from build123d import *

# Parameters (mm, degrees)
F0_W     = 15
F0_H     = 10
F0_R     = 2
F1_DEPTH = 8.5
F2_W     = 2.25
F2_H     = 3.4951120354
F3_DEPTH = 25
F4_DEPTH = 6.5


with BuildPart() as f1:
    # F0 (on Top) → F1 (new body)
    with BuildSketch(Plane.XY):
        Rectangle(F0_W, F0_H)
        Circle(F0_R, mode=Mode.SUBTRACT)
    extrude(amount=F1_DEPTH)

    # F2 (on face) → F3 (cut)
    with BuildSketch(Plane.YZ.offset(7.5)):
        Polygon((5, 3), (2, 0), (5, 0), align=None)
        with Locations((3.875, 4.7475560177)):
            Rectangle(F2_W, F2_H)
        with Locations((-3.875, 4.7475560177)):
            Rectangle(F2_W, F2_H)
        Polygon((-5, 0), (-2, 0), (-5, 3), align=None)
    extrude(amount=-F3_DEPTH, mode=Mode.SUBTRACT)

    # F4 (cut): faces of the model
    f4_faces = [f1.faces().sort_by_distance(p)[0] for p in [
        (4.5185944257, 0, 0),
        (-4.5185944257, 0, 0),
    ]]
    extrude(f4_faces, amount=-F4_DEPTH, mode=Mode.SUBTRACT)


solid = f1.part
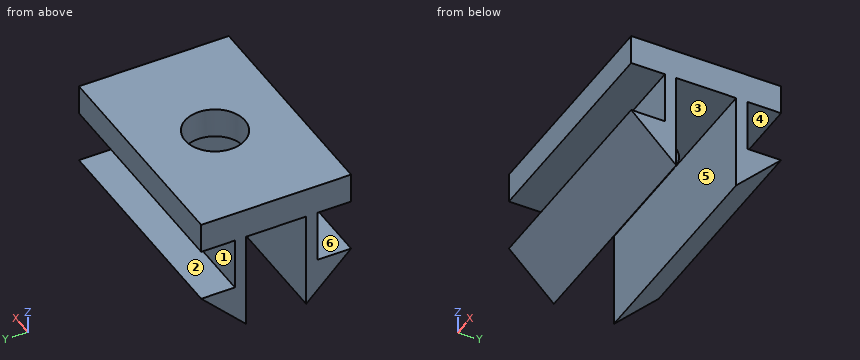
Here's how the part is built. I have some questions about the finished solid (model axes, mm). Face numbers are marked on the shaded views. A direction names the side the tool comes from. Coordinates: 2 decimals unless noted, no trailing zeros. Write each loop counter-clockwise with the first axis right and the second up, starting at its lowest first coordinate (ties: lowest second). Pieces come first, ordered by that corner, then holes.
Item 1: On a 3-axis mill with a long thin cutter (end or side, diameter ignored), from which of +Z, -Z, +X, -X, +Y, -Y can I reach the whole of each face in a straight line? I mean the marked faces 4, 5 and 6. Say none if no direction works.
Item 2: If I drill on line 1 (Y direction, x = 5.75, z = 5); line 2 (X direction, y = 0, z = 7); line 3 (Y direction, x = 0, z = 7.9), over which ranges is the centre line in solid material (lowest first)?
Item 3: I want a section at C-C on x = 1.5. Write out the boundary of the cut face in (y, z), and give its area (3 significant figures).
Item 4: I want a section at D-D on z = 7. Write out the boundary of the cut face in (x, y), and give its area (3 significant figures).
Item 5: If we mould it in two halves opening along Y, with no side actions, what happens to the marked faces 1, 2 and 3? For each: +Y half, -Y half, draft (parallel to the pull), parting line (faces both ways), or undercut.
Item 6: Will these pins go through, and if not, where does the flat tip stop? pin 1 (4 mm diameter, centred on x = -1, z = 5.5, fed in from -Y); pin 2 (1.1 mm diameter, centred on x = -0.5, y = 4, fed in from -Z); pin 3 (0.7 mm diameter, centred on x = -1.5, y = -4, fed in from -Z); pin 4 (5 mm diameter, centred on x = -1.5, z = 2.5, fed in from +Y).
Item 7: I want a section at B-B on y = 0. Write out the boundary of the cut face in (x, z), and give its area (3 significant figures).
Item 8: I want a section at A-A on z = 5. Write out the boundary of the cut face in (x, y), and give its area (3 significant figures).
Findings below:
1. face 4: +X, -X, +Y
1. face 5: -Z, +X, -X
1. face 6: +X, -X, -Y
2. line 1: y = -2.75 to -2, 2 to 2.75
2. line 2: x = -7.5 to -2, 2 to 7.5
2. line 3: y = -5 to -2, 2 to 5
3. outline: (-5, 3) - (-2, 0) - (-2, 6.5) - (-1.32, 6.5) - (-1.32, 8.5) - (-5, 8.5) - (-5, 6.5) - (-2.75, 6.5) - (-2.75, 3) - close; (1.32, 6.5) - (2, 6.5) - (2, 0) - (5, 3) - (2.75, 3) - (2.75, 6.5) - (5, 6.5) - (5, 8.5) - (1.32, 8.5) - close
3. area: 29.0 mm2
4. outline: (-7.5, -5) - (7.5, -5) - (7.5, 5) - (-7.5, 5) - close; hole circle Ø4 at (0, 0)
4. area: 137 mm2
5. face 1: +Y half
5. face 2: draft
5. face 3: undercut
6. pin 1: stops at y = -5
6. pin 2: stops at z = 1.45
6. pin 3: stops at z = 1.65
6. pin 4: stops at y = 5
7. outline: (-7.5, 6.5) - (-2, 6.5) - (-2, 8.5) - (-7.5, 8.5) - close; (2, 6.5) - (7.5, 6.5) - (7.5, 8.5) - (2, 8.5) - close
7. area: 22.0 mm2
8. outline: (-7.5, -2.75) - (7.5, -2.75) - (7.5, -2) - (-7.5, -2) - close; (-7.5, 2) - (7.5, 2) - (7.5, 2.75) - (-7.5, 2.75) - close
8. area: 22.5 mm2
